from build123d import *

# Parameters (mm, degrees)
EXTRUDE_1_DEPTH = 3.4
EXTRUDE_START   = -0.6
SKETCH_2_R      = 2.4
SKETCH_2_R_2    = 1.2
EXTRUDE_2_DEPTH = 0.6
CHAMFER_1_SIZE  = 0.2


with BuildPart() as part:
    # 草图1 → 凸台-拉伸1 (new body)
    with BuildSketch(Plane(origin=(0, 0, 0), x_dir=(0, 0, -1), z_dir=(1, 0, 0))):
        with BuildLine():
            Line((1.326649916, 2), (3.919183588, 2))
            ThreePointArc((3.919183588, 2), (0, 4.4), (-3.919183588, 2))
            Line((-3.919183588, 2), (-1.326649916, 2))
            ThreePointArc((-1.326649916, 2), (0, 2.4), (1.326649916, 2))
        make_face()
        with BuildLine():
            ThreePointArc((4.4, 0), (4.278107513, 1.028492151), (3.919183588, 2))
            Line((3.919183588, 2), (1.326649916, 2))
            ThreePointArc((1.326649916, 2), (2.114705629, 1.134909732), (2.4, 0))
            ThreePointArc((2.4, 0), (2.114705629, -1.134909732), (1.326649916, -2))
            Line((1.326649916, -2), (3.919183588, -2))
            ThreePointArc((3.919183588, -2), (4.278107513, -1.028492151), (4.4, 0))
        make_face()
        with BuildLine():
            Line((-1.326649916, 2), (-3.919183588, 2))
            ThreePointArc((-3.919183588, 2), (-4.4, 0), (-3.919183588, -2))
            Line((-3.919183588, -2), (-1.326649916, -2))
            ThreePointArc((-1.326649916, -2), (-2.4, 0), (-1.326649916, 2))
        make_face()
        with BuildLine():
            ThreePointArc((-3.919183588, -2), (-4.4, 0), (-3.919183588, 2))
            Line((-3.919183588, 2), (-10, 2))
            Line((-10, 2), (-10, -2))
            Line((-10, -2), (-3.919183588, -2))
        make_face()
        with BuildLine():
            Line((10, -2), (10, 2))
            Line((10, 2), (3.919183588, 2))
            ThreePointArc((3.919183588, 2), (4.278107513, 1.028492151), (4.4, 0))
            ThreePointArc((4.4, 0), (4.278107513, -1.028492151), (3.919183588, -2))
            Line((3.919183588, -2), (10, -2))
        make_face()
        with BuildLine():
            ThreePointArc((-3.919183588, -2), (0, -4.4), (3.919183588, -2))
            Line((3.919183588, -2), (1.326649916, -2))
            ThreePointArc((1.326649916, -2), (0, -2.4), (-1.326649916, -2))
            Line((-1.326649916, -2), (-3.919183588, -2))
        make_face()
    extrude(amount=EXTRUDE_1_DEPTH)

    # 草图2 → 凸台-拉伸2 (add)
    with BuildSketch(Plane(origin=(3.4, 0, 0), x_dir=(0, 0, -1), z_dir=(1, 0, 0)).offset(EXTRUDE_START)):
        Circle(SKETCH_2_R)
        Circle(SKETCH_2_R_2, mode=Mode.SUBTRACT)
    extrude(amount=EXTRUDE_2_DEPTH)

    # 倒角1
    chamfer_1_edges = [part.edges().sort_by_distance(p)[0] for p in [
        (0, 2, 1.326649916),
    ]]
    chamfer(chamfer_1_edges, length=CHAMFER_1_SIZE)


solid = part.part
Can you work these out from the model? Positions are in its coordinate system, mm. A direction names the side the tool comes from. Coordinates: 2 decimals unless noted, no trailing zeros. Loops run counter-clockwise (first coordinate to the right, second up) from the corner with the lowest first, then second, coordinate; pieces in that order, holes last. Notation, with made-up numbers: M 12.5,57.5 L 70.5,57.5 A22 cw 70.5,86.5 Z; hole C -35.75,36 d11. An arc over 180 degrees is marked long. Answer as CSV lines item,"result". Start each with the question number.
1. For pin 1 Ø4 at (y, z) = (0, 0) entering from +X; pin 2 Ø1.7 at (x, z) = (1, 8) entering from -Y; pin 3 Ø1 at (y, z) = (3.5, -6) entering from -X, each with a flat end and sliding along its axis, tell me the tip position at first contact or that it passes through.
2. If I drill on probe 1 along Y at (x, z) = (1.75, 4.75); probe 2 along Z at (x, y) = (1.1, -1.5); probe 3 along Z at (x, y) = (0.4, -0.5), over which ranges is the centre line in solid material (lowest first)? Write a range as [from, to].
3. Suppose I cut it at C-C, the plane y = -3.25. List the corners of the cut face in (x, z) for me, plus the area to 3 significant figures.
4. Thinking about a two-plate mould opening in Z: for faces 1 (the face through (2.8, 1, 1)), 2 (the face through (2, 2, 7)), 3 (the face through (1.7, 4.4, -0.1)), which applies, +Z half, -Z half, draft (parallel to the pull), parting line (faces both ways), or undercut?
5. Suppose I cut it at A-A, the plane z = 0. List the corners of the cut face in (x, y) for me.
6. For faces 4 (the face through (2, 2, -7)), 5 (the face through (1.7, -4.4, 0.1)), 6 (the face through (3.4, -2, 0)), 7 (the face through (2, -2, -7)), 8 (the face through (2, -2, 7)), which set-ups out of +Z, -Z, +X, -X, +Y, -Y let a thin tool reach every point of the face, with its end or its side?
7. Suppose I cut it at D-D, the plane z = -5. List the corners of the cut face in (x, y) for me.
8. Suppose I cut it at B-B, the plane x = 1.95. List the corners of the cut face in (y, z) for me, plus the area to 3 significant figures.
Output:
1,pin 1,"stops at x = 3.4"
1,pin 2,"stops at y = -2"
1,pin 3,"passes through"
2,probe 1,"y = [-2, 2]"
2,probe 2,"z = [-10, -1.87], [1.87, 10]"
2,probe 3,"z = [-10, -2.35], [2.35, 10]"
3,outline,"M 0,-2.97 L 3.4,-2.97 L 3.4,2.97 L 0,2.97 Z"
3,area,"20.2 mm^2"
4,face 1,"undercut"
4,face 2,"draft"
4,face 3,"parting line"
5,outline,"M 0,-4.4 L 3.4,-4.4 L 3.4,-1.2 L 2.8,-1.2 L 2.8,-2.4 L 0.2,-2.4 L 0,-2.6 Z; M 0,2.6 L 0.2,2.4 L 2.8,2.4 L 2.8,1.2 L 3.4,1.2 L 3.4,4.4 L 0,4.4 Z"
6,face 4,"-Z, +X, -X, +Y"
6,face 5,"+X, -X, -Y"
6,face 6,"+Z, -Z, +X, +Y, -Y"
6,face 7,"-Z, +X, -X, -Y"
6,face 8,"+Z, +X, -X, -Y"
7,outline,"M 0,-2 L 3.4,-2 L 3.4,2 L 0,2 Z"
8,outline,"M -2,-10 L 2,-10 L 2,-3.92 A4.4 ccw 2,3.92 L 2,10 L -2,10 L -2,3.92 A4.4 ccw -2,-3.92 Z; hole C 0,0 d4.8"
8,area,"88.8 mm^2"
